Check sheet for the modelled part. Datum: model origin and axes. Units: mm. A direction names the side the tool comes from. Coordinates: 2 decimals unless noted, no trailing zeros. Loops run counter-clockwise (first coordinate to the right, second up) from the corner with the lowest first, then second, coordinate; pieces in that order, holes last. Notation, with made-up numbers: (-16, -8.5) -> (-5, -8.5) arc R10 ccw to (-5, -1.5) -> close; hole circle Ø10 at (41.5, -13). An arc over 180 degrees is marked (long way). Use one line per item in the form item = value.
from build123d import *

# Parameters (mm, degrees)
F0_R     = 45
F1_DEPTH = 12.7
F3_DEPTH = 25.401
F4_R     = 25.00625
F5_DEPTH = 25.401
F6_R     = 1.5875
F7_DEPTH = 50.8


# Not quite as in the source:
# - a feature names something its author has since deleted; it is built from what else it names


with BuildPart() as f1:
    # F0 (on Front) → F1 (new body, symmetric)
    with BuildSketch(Plane.XZ):
        Circle(F0_R)
    extrude(amount=F1_DEPTH, both=True)

    # F2 (on face) → F3 (cut, through all)
    with BuildSketch(Plane.XZ.offset(12.7)):
        with BuildLine():
            Line((-33.3949635986, 30.1625), (33.3949635986, 30.1625))
            ThreePointArc((33.3949635986, 30.1625), (0, 45), (-33.3949635986, 30.1625))
        make_face()
        with BuildLine():
            ThreePointArc((-33.3949635986, -30.1625), (0, -45), (33.3949635986, -30.1625))
            Line((33.3949635986, -30.1625), (-33.3949635986, -30.1625))
        make_face()
    extrude(amount=-F3_DEPTH, mode=Mode.SUBTRACT)

    # F4 (on face) → F5 (cut, through all)
    with BuildSketch(Plane.XZ.offset(12.7)):
        Circle(F4_R)
    extrude(amount=-F5_DEPTH, mode=Mode.SUBTRACT)

    # F6 (on face) → F7 (cut)
    with BuildSketch(Plane.XY.offset(30.1625)):
        with Locations((30.2199635986, 0)):
            Circle(F6_R)
        Circle(F6_R)
        with Locations((-30.2199635986, 0)):
            Circle(F6_R)
    extrude(amount=-F7_DEPTH, mode=Mode.SUBTRACT)


solid = f1.part
(1) Scan lines: line 1 along Z through (x, y) = (0, 5.5); line 2 along Y through (x, z) = (0, 28.55); line 3 along X through (y, z) = (1.25, -17). Record each from-to range of solid material in increasing order.
Established:
line_1 = -30.16 to -25.01, 25.01 to 30.16
line_2 = -12.7 to -1.59, 1.59 to 12.7
line_3 = -41.67 to -31.2, -29.24 to -18.34, 18.34 to 29.24, 31.2 to 41.67
(2) Section check C-C, the plane y = 10. Record the boundary of the cut face in (x, z), plus the area to 3 significant figures.
Established:
outline = (-33.39, -30.16) -> (33.39, -30.16) arc R45 ccw to (33.39, 30.16) -> (-33.39, 30.16) arc R45 ccw to start; hole circle Ø50.01 at (0, 0)
area = 3,030 mm²
(3) Tool access check on faces 1 (the flat face through (0, 0, -30.162)), 2 (the flat face through (-30, 0, -20.637)). Record the directions out of +Z, -Z, +X, -X, +Y, -Y that give a thin tool (end or side, any length) a straight path to the whole face; none if there is none.
Established:
face_1 = -Z, +X, -X, +Y, -Y
face_2 = +Z
(4) Section check A-A, the plane z = 0. Record the boundary of the cut face in (x, y) (1 decimal).
Established:
outline = (-45, -12.7) -> (-25, -12.7) -> (-25, 12.7) -> (-45, 12.7) -> close; (25, -12.7) -> (45, -12.7) -> (45, 12.7) -> (25, 12.7) -> close; hole circle Ø3.2 at (-30.2, 0); hole circle Ø3.2 at (30.2, 0)
(5) Mould release check, pull along Y, two halves, no side actions. Record for faces 3 (the flat face through (0, -3, 30.162)), 4 (the flat face through (-1, 12.7, -26)), 5 (the flat face through (30, 0, -20.637)): +Y half, -Y half, draft (parallel to the pull), parting line (faces both ways), or undercut.
Established:
face_3 = draft
face_4 = +Y half
face_5 = undercut
(6) Section check D-D, the plane y = 0. Record the boundary of the cut face in (x, z).
Established:
outline = (-33.39, -30.16) -> (33.39, -30.16) arc R45 ccw to (33.39, 30.16) -> (31.81, 30.16) -> (31.81, -20.64) -> (28.63, -20.64) -> (28.63, 30.16) -> (1.59, 30.16) -> (1.59, 24.96) arc R25.01 cw (long way) to (-1.59, 24.96) -> (-1.59, 30.16) -> (-28.63, 30.16) -> (-28.63, -20.64) -> (-31.81, -20.64) -> (-31.81, 30.16) -> (-33.39, 30.16) arc R45 ccw to start
(7) Section check B-B, the plane x = 0. Record the boundary of the cut face in (y, z).
Established:
outline = (-12.7, -30.16) -> (12.7, -30.16) -> (12.7, -25.01) -> (-12.7, -25.01) -> close; (-12.7, 25.01) -> (-1.59, 25.01) -> (-1.59, 30.16) -> (-12.7, 30.16) -> close; (1.59, 25.01) -> (12.7, 25.01) -> (12.7, 30.16) -> (1.59, 30.16) -> close
(8) Go/stop test with flat-tipped pins: P1, Ø4, axis at y = 0.5, z = -11.5, coming from the -X side; P2, Ø1.6, axis at x = 30.5, y = -0.5, coming from the +Z side; P3, Ø4, axis at y = 2, z = -23, coming from the +X side. Record where each tip stops, or that it passes through.
Established:
P1 = -43.99
P2 = -20.64
P3 = 39.8
